Geometry check sheet. Reference: the model listing, model coordinates, mm. Face numbers are marked on the shaded views. A direction names the side the tool comes from. Coordinates: 2 decimals unless noted, no trailing zeros. Write each loop counter-clockwise with the first axis right and the second up, starting at its lowest first coordinate (ties: lowest second). Pieces come first, ordered by that corner, then holes.
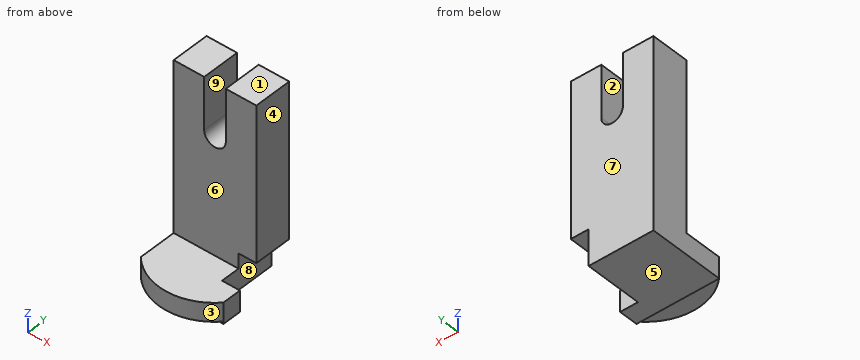
from build123d import *

# Parameters (mm, degrees)
F0_W      = 55.3297251463
F0_H      = 127.18950212
F1_DEPTH  = 25.4
F2_W      = 7.2318934835
F2_H      = 34.8967574537
F3_DEPTH  = 25.4
F5_DEPTH  = 25.4
F6_W      = 55.3297251463
F6_H      = 14.0431076288
F7_DEPTH  = 25.4
F9_DEPTH  = 12.446
F10_W     = 25.4
F10_H     = 24.0572243929
F11_DEPTH = 11.938
F12_W     = 11.938
F12_H     = 12.7
F13_DEPTH = 25.4


with BuildPart() as f1:
    # F0 (on Front) → F1 (new body)
    with BuildSketch(Plane.XZ):
        Rectangle(F0_W, F0_H)
    extrude(amount=-F1_DEPTH)

    # F2 (on face) → F3 (cut)
    with BuildSketch(Plane.XZ):
        with Locations((-3.6159467418, 46.1463723332)):
            Rectangle(F2_W, F2_H)
        with Locations((3.6159467418, 46.1463723332)):
            Rectangle(F2_W, F2_H)
    extrude(amount=-F3_DEPTH, mode=Mode.SUBTRACT)

    # F4 (on face) → F5 (cut)
    with BuildSketch(Plane(origin=(0, 25.4, 0), x_dir=(-1, 0, 0), z_dir=(0, 1, 0))):
        with BuildLine():
            Line((7.2318934835, 28.6979936063), (-7.2318934835, 28.6979936063))
            ThreePointArc((-7.2318934835, 28.6979936063), (0, 21.4661001228), (7.2318934835, 28.6979936063))
        make_face()
    extrude(amount=-F5_DEPTH, mode=Mode.SUBTRACT)

    # F6 (on face) → F7 (join)
    with BuildSketch(Plane.XZ):
        with Locations((0, -56.5731972456)):
            Rectangle(F6_W, F6_H)
    extrude(amount=F7_DEPTH)

    # F8 (on face) → F9 (join)
    with BuildSketch(Plane.XY.offset(-49.5516434312)):
        with BuildLine():
            Line((27.6648625731, -25.4), (-27.6648625731, -25.4))
            ThreePointArc((-27.6648625731, -25.4), (0, -37.6812428416), (27.6648625731, -25.4))
        make_face()
    extrude(amount=-F9_DEPTH)

    # F10 (on face) → F11 (cut)
    with BuildSketch(Plane.YZ.offset(27.6648625731)):
        with Locations((12.7, -51.5661388636)):
            Rectangle(F10_W, F10_H)
    extrude(amount=-F11_DEPTH, mode=Mode.SUBTRACT)

    # F12 (on face) → F13 (cut)
    with BuildSketch(Plane.XY.offset(-49.5516434312)):
        with Locations((21.6958625731, -6.35)):
            Rectangle(F12_W, F12_H)
    extrude(amount=-F13_DEPTH, mode=Mode.SUBTRACT)


solid = f1.part
1. Sectioned sample at A-A, the plane y = 17. Record the boundary of the cut face in (x, z), and give its area (3 significant figures).
Computed values:
outline: (-27.66, -63.59) - (15.73, -63.59) - (15.73, -39.54) - (27.66, -39.54) - (27.66, 63.59) - (7.23, 63.59) - (7.23, 28.7) arc R7.23 cw to (-7.23, 28.7) - (-7.23, 63.59) - (-27.66, 63.59) - close
area: 6,160 mm2
2. Sectioned sample at B-B, the plane x = 0. Record the boundary of the cut face in (y, z), and give its area (3 significant figures).
Computed values:
outline: (-37.68, -62) - (-25.4, -62) - (-25.4, -63.59) - (25.4, -63.59) - (25.4, 21.47) - (0, 21.47) - (0, -49.55) - (-37.68, -49.55) - close
area: 2,670 mm2
3. Draft check along X on the marked faces 1, 2, 3 and 4. Enter one of: released by +X, released by -X, zero draft, split by the parting line, or undercut.
Computed values:
face 1: zero draft
face 2: undercut
face 3: split by the parting line
face 4: released by +X
4. Sectioned sample at C-C, the plane z = -45. Record the boundary of the cut face in (x, y).
Computed values:
outline: (-27.66, 0) - (15.73, 0) - (15.73, 25.4) - (-27.66, 25.4) - close
5. Thickness scan on line 1 along Y through (x, z) = (8, -24); line 2 along Z through (x, y) = (-17, -6); line 3 along X through (y, z) = (0.5, -54.5). Record the ranges inside material, lowest first.
Computed values:
line 1: y = 0 to 25.4
line 2: z = -63.59 to -49.55
line 3: x = -27.66 to 15.73
6. Gauge pin test, flat ends, axial feed: pin 1 Ø1 at (x, z) = (-6.5, -11) entering from -Y; pin 2 Ø0.8 at (x, z) = (-6.5, -63) entering from -Y; pin 3 Ø1 at (x, y) = (-5.5, 2.5) entering from +Z. Record the tip position at first contact, or that the pin passes through.
Computed values:
pin 1: stops at y = 0
pin 2: stops at y = -25.4
pin 3: stops at z = 24.66
7. Access from +Z, -Z, +X, -X, +Y, -Y to the whole of each face (thin tool, end or side, straight path). Record for the marked faces 5, 6, 7, 8 and 9.
Computed values:
face 5: -Z, +X, -X, +Y, -Y
face 6: +Z, +X, -X, -Y
face 7: +Z, -Z, +X, -X, +Y
face 8: -Z, +X, +Y
face 9: +Z, +Y, -Y
8. Sectioned sample at D-D, the plane x = -14. Record the boundary of the cut face in (y, z).
Computed values:
outline: (-34.95, -62) - (-25.4, -62) - (-25.4, -63.59) - (25.4, -63.59) - (25.4, 63.59) - (0, 63.59) - (0, -49.55) - (-34.95, -49.55) - close
